Part model, mm, in its own coordinate system. Face numbers are marked on the shaded views. A direction names the side the tool comes from. Round coordinates to 2 decimals unless told otherwise and drop trailing zeros. Loops run counter-clockwise (first coordinate to the right, second up) from the corner with the lowest first, then second, coordinate; pieces in that order, holes last.
1) Probe line 1 (Y direction, x = -280, z = 166.5); line 2 (Y direction, x = -18, z = 122.5); line 3 (Y direction, x = 0, z = 29.5). List the from-to ranges inside material, lowest first.
2) Drop flat-ended pins along their axis: P1, Ø2, axis at y = 533.5, z = 30, coming from the -X side; P2, Ø10, axis at y = -647, z = 112, coming from the +X side; P3, Ø1, axis at x = -127, z = 27.5, coming from the +Y side. Give the stop position or say it passes through.
3) Mould opens along X. For the marked faces 1, 2 and 3 say: +X half, -X half, draft (parallel to the pull), parting line (faces both ways), or undercut.
4) Band-saw the part on B-B, the plane x = -280. Write the cut outline in (y, z).
5) Band-saw the part on C-C, the plane z = 33.5. State how many separate pieces and enclosed holes the cut face has, then the cut area to 3 significant figures.
6) Band-saw the part on A-A, the plane y = 0. Write the cut outline in (x, z), then the cut area to 3 significant figures.
7) 3-axis set-ups, long thin cutter, end or side, ignore diameter. For the marked faces 4, 5, 6, 7 and 8: which of +Z, -Z, +X, -X, +Y, -Y reach the whole face in a straight line?
8) Band-saw the part on D-D, the plane y = -400. Write the cut outline in (x, z), then the cut area to 3 significant figures.
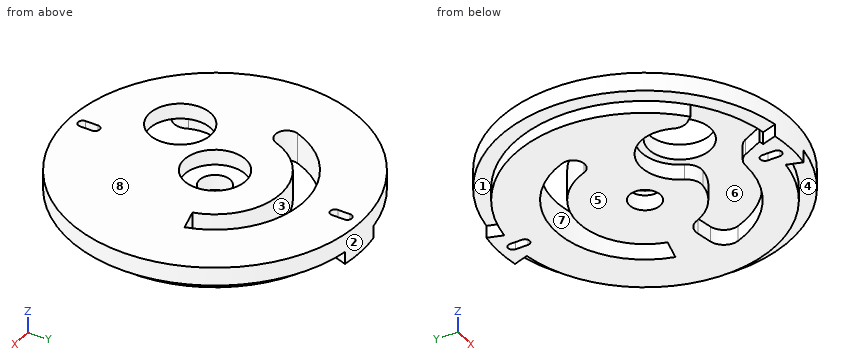
from build123d import *

# Parameters (mm, degrees)
ESQUISSE1_R             = 950
ESQUISSE1_R_2           = 100
ESQUISSE1_R_3           = 200
BOSS_EXTRU_2_DEPTH      = 200
ESQUISSE4_R             = 200
ENL_V_MAT_EXTRU_2_DEPTH = 100
ESQUISSE5_R             = 200
ENL_V_MAT_EXTRU_3_DEPTH = 100
ENL_V_MAT_EXTRU_4_DEPTH = 80


with BuildPart() as part:
    # Esquisse1 → Boss.-Extru.2 (new body)
    with BuildSketch(Plane.XY):
        Circle(ESQUISSE1_R)
        Circle(ESQUISSE1_R_2, mode=Mode.SUBTRACT)
        with Locations((-280, -400)):
            Circle(ESQUISSE1_R_3, mode=Mode.SUBTRACT)
        with BuildLine():
            Line((30, -780), (30, -860))
            ThreePointArc((30, -860), (0, -890), (-30, -860))
            Line((-30, -860), (-30, -780))
            ThreePointArc((-30, -780), (0, -750), (30, -780))
        make_face(mode=Mode.SUBTRACT)
        with BuildLine():
            Line((415.348105304, 111.292189394), (560.236979248, 150.115046159))
            ThreePointArc((560.236979248, 150.115046159), (25.299244672, 579.447968517), (-545.021720056, 198.371683129))
            ThreePointArc((-545.021720056, 198.371683129), (-500.196284246, 102.243225821), (-404.067826938, 147.06866163))
            ThreePointArc((-404.067826938, 147.06866163), (18.756336567, 429.59073528), (415.348105304, 111.292189394))
        make_face(mode=Mode.SUBTRACT)
        with BuildLine():
            Line((30, 780), (30, 860))
            ThreePointArc((30, 860), (0, 890), (-30, 860))
            Line((-30, 860), (-30, 780))
            ThreePointArc((-30, 780), (0, 750), (30, 780))
        make_face(mode=Mode.SUBTRACT)
    extrude(amount=BOSS_EXTRU_2_DEPTH)

    # Esquisse4 → Enlèv. mat.-Extru.2 (cut)
    with BuildSketch(Plane.XY.offset(200)):
        Circle(ESQUISSE4_R)
    extrude(amount=-ENL_V_MAT_EXTRU_2_DEPTH, mode=Mode.SUBTRACT)

    # Esquisse5 → Enlèv. mat.-Extru.3 (cut)
    with BuildSketch(Plane(origin=(0, 0, 0), x_dir=(-1, 0, 0), z_dir=(0, 0, -1))):
        with BuildLine():
            ThreePointArc((201.863253444, -825.682279638), (390.762908215, -754.853859739), (557.650174642, -641.503143189))
            Line((557.650174642, -641.503143189), (525.236890093, -604.21592467))
            ThreePointArc((525.236890093, -604.21592467), (501.276797335, -549.262070437), (513.052344937, -490.479856982))
            ThreePointArc((513.052344937, -490.479856982), (380.433331839, -171.060824987), (55.598868761, -289.799581223))
            ThreePointArc((55.598868761, -289.799581223), (12.641866668, -335.439232515), (-49.041983374, -346.547087517))
            ThreePointArc((-49.041983374, -346.547087517), (-213.58758579, -277.273048088), (-322.558312447, -135.853358705))
            ThreePointArc((-322.558312447, -135.853358705), (-366.878979382, -86.853774186), (-432.082648055, -76.187828748))
            Line((-432.082648055, -76.187828748), (-532.616227494, -93.91461127))
            ThreePointArc((-532.616227494, -93.91461127), (-602.060758652, -142.755312647), (-608.933484223, -227.376365948))
            ThreePointArc((-608.933484223, -227.376365948), (-372.346828507, -532.783107184), (-4.23006723, -649.986235648))
            ThreePointArc((-4.23006723, -649.986235648), (48.386746731, -665.352188625), (84.998557826, -706.147003376))
            Line((84.998557826, -706.147003376), (148.761821167, -836.881067155))
            ThreePointArc((148.761821167, -836.881067155), (175.401935414, -831.705573537), (201.863253444, -825.682279638))
        make_face()
        with Locations((280, -400)):
            Circle(ESQUISSE5_R, mode=Mode.SUBTRACT)
    extrude(amount=-ENL_V_MAT_EXTRU_3_DEPTH, mode=Mode.SUBTRACT)

    # Esquisse6 → Enlèv. mat.-Extru.4 (cut)
    with BuildSketch(Plane(origin=(0, 0, 0), x_dir=(-1, 0, 0), z_dir=(0, 0, -1))):
        with BuildLine():
            Line((-118.297135816, 841.72785843), (-149.624359786, 938.143139909))
            ThreePointArc((-149.624359786, 938.143139909), (-950, 0), (-149.624359786, -938.143139909))
            Line((-149.624359786, -938.143139909), (-118.297135816, -841.72785843))
            ThreePointArc((-118.297135816, -841.72785843), (-850, 0), (-118.297135816, 841.72785843))
        make_face()
        with BuildLine():
            Line((118.297135816, 841.72785843), (149.624359786, 938.143139909))
            ThreePointArc((149.624359786, 938.143139909), (950, 0), (149.624359786, -938.143139909))
            Line((149.624359786, -938.143139909), (118.297135816, -841.72785843))
            ThreePointArc((118.297135816, -841.72785843), (850, 0), (118.297135816, 841.72785843))
        make_face()
    extrude(amount=-ENL_V_MAT_EXTRU_4_DEPTH, mode=Mode.SUBTRACT)


solid = part.part
Reported:
1. line 1: y = -907.8 to -600, -200 to 326.34, 507.94 to 907.8
1. line 2: y = -949.83 to -884, -756 to -199.19, 199.19 to 429.62, 579.72 to 756, 884 to 949.83
1. line 3: y = -950 to -890, -750 to -650.1, -341.2 to -100, 100 to 430, 580 to 750, 890 to 950
2. P1: stops at x = -662.53
2. P2: stops at x = 700.24
2. P3: stops at y = 941.54
3. face 1: draft
3. face 2: parting line
3. face 3: undercut
4. outline: (-907.8, 80) - (-802.56, 80) - (-802.56, 100) - (-600, 100) - (-600, 200) - (-907.8, 200) - close; (-200, 100) - (-150, 100) - (-150, 0) - (326.34, 0) - (326.34, 200) - (-200, 200) - close; (507.94, 0) - (802.56, 0) - (802.56, 80) - (907.8, 80) - (907.8, 200) - (507.94, 200) - close
5. separate pieces: 1
5. enclosed holes: 4
5. area: 1,590,000 mm2
6. outline: (-950, 80) - (-850, 80) - (-850, 0) - (-100, 0) - (-100, 100) - (-200, 100) - (-200, 200) - (-950, 200) - close; (100, 0) - (850, 0) - (850, 80) - (950, 80) - (950, 200) - (200, 200) - (200, 100) - (100, 100) - close
6. area: 304,000 mm2
7. face 4: -Z, +X
7. face 5: -Z, +X, -X, +Y, -Y
7. face 6: -Z
7. face 7: +Z, -Z
7. face 8: +Z, +X, -X, +Y, -Y
8. outline: (-861.68, 80) - (-750, 80) - (-750, 0) - (-530, 0) - (-530, 100) - (-480, 100) - (-480, 200) - (-861.68, 200) - close; (-80, 100) - (512.35, 100) - (512.35, 0) - (750, 0) - (750, 80) - (861.68, 80) - (861.68, 200) - (-80, 200) - close
8. area: 183,000 mm2
